```python
from build123d import *

# Parameters (mm, degrees)
SKETCH_1_W          = 42.7
SKETCH_1_H          = 33
EXTRUDE_1_DEPTH     = 4
SKETCH_2_R          = 1.5
SKETCH_2_W          = 10
SKETCH_2_H          = 4
SKETCH_2_W_2        = 4
SKETCH_2_H_2        = 14
CUT_EXTRUDE_2_DEPTH = 4


with BuildPart() as part:
    # Эскиз1 → Бобышка-Вытянуть1 (new body)
    with BuildSketch(Plane.XY):
        with Locations((17.35, 12.5)):
            Rectangle(SKETCH_1_W, SKETCH_1_H)
    extrude(amount=EXTRUDE_1_DEPTH)

    # Эскиз2 → Вырез-Вытянуть2 (cut)
    with BuildSketch(Plane.XY.offset(4)):
        with Locations((12.35, 12.5)):
            Circle(SKETCH_2_R)
        with Locations(Location((22.35, 12.5, 0), (0, 0, 180))):
            Circle(SKETCH_2_R)
        with Locations((9.85, 27)):
            Rectangle(SKETCH_2_W, SKETCH_2_H)
        with Locations((24.85, 27)):
            Rectangle(SKETCH_2_W, SKETCH_2_H)
        with Locations((-2, 3)):
            Rectangle(SKETCH_2_W_2, SKETCH_2_H_2)
        with Locations((-2, 22)):
            Rectangle(SKETCH_2_W_2, SKETCH_2_H_2)
        with Locations((24.85, -2)):
            Rectangle(SKETCH_2_W, SKETCH_2_H)
        with Locations((9.85, -2)):
            Rectangle(SKETCH_2_W, SKETCH_2_H)
        with Locations((36.7, 3)):
            Rectangle(SKETCH_2_W_2, SKETCH_2_H_2)
        with Locations((36.7, 22)):
            Rectangle(SKETCH_2_W_2, SKETCH_2_H_2)
    extrude(amount=-CUT_EXTRUDE_2_DEPTH, mode=Mode.SUBTRACT)


solid = part.part
```
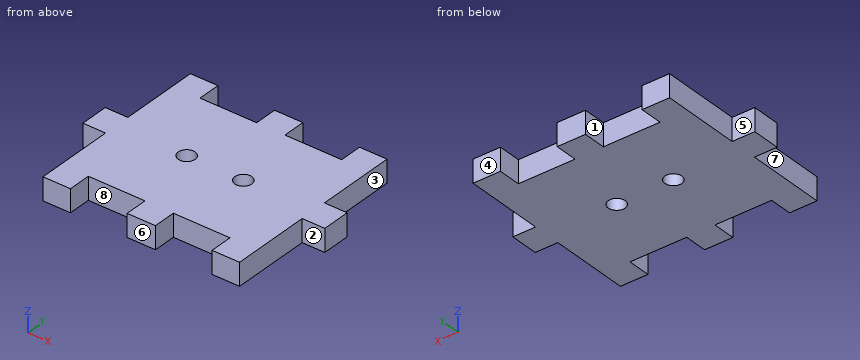
Geometry: final body of the model. Coordinates: model frame, mm. Face numbers are marked on the shaded views. A direction names the side the tool comes from. Coordinates: 2 decimals unless noted, no trailing zeros. Loops run counter-clockwise (first coordinate to the right, second up) from the corner with the lowest first, then second, coordinate; pieces in that order, holes last. Notation, with made-up numbers: (23.25, 49) -> (42.25, 49) arc R16 ccw to (42.25, 56) -> close; hole circle Ø8 at (37.25, 27.5). An arc over 180 degrees is marked (long way). Use a Markdown table: item, result. Add a question column.
(1) Pin query (flat end, axial travel): pin 1 Ø2 at (y, z) = (24.5, 2.5) entering from -X; pin 2 Ø2 at (x, z) = (24.5, 1.5) entering from -Y; pin 3 Ø1.2 at (x, z) = (25, 2) entering from +Y. Return the tip coordinate at first contact, or that it passes through.
(2) Section query D-D, the plane x = 8. Return loops of the section in (y, z), plus the area to 3 significant figures.
(3) Access query for the marked faces 4, 5, 6, 7 and 8. Directions: +Z, -Z, +X, -X, +Y, -Y. A direction counts if a zero-diameter tool reaches every point of the face in a straight line with its end or side. Return the directions, or none.
(4) Section query C-C, the plane z = 2.15. State how many separate pieces and enclosed holes the cut face has, plus the area to 3 significant figures.
(5) Mould query, pull axis X, two halves, no side actions, for the marked faces 1, 2 and 3. Classes: pulls with the +X half, pulls with the -X half, needs draft (parallel to the pull), parting line crosses it, or undercut.
(6) Section query A-A, the plane y = 12.5. Return loops of the section in (x, z), plus the area to 3 significant figures.
(7) Line query: line 1 along X through (y, z) = (26, 0.45); line 2 along Y through (x, z) = (12.35, 1.65); line 3 along Y through (x, z) = (28.5, 2). Output: solid intervals per line, ascending.
(8) Section query B-B, the plane x = 12.35. Return loops of the section in (y, z).
Answer:
| question | item | result |
|---|---|---|
| 1 | pin 1 | stops at x = 0 |
| 1 | pin 2 | stops at y = 0 |
| 1 | pin 3 | stops at y = 25 |
| 2 | outline | (0, 0) -> (25, 0) -> (25, 4) -> (0, 4) -> close |
| 2 | area | 100 mm^2 |
| 3 | face 4 | +Z, -Z, +X, -X, +Y |
| 3 | face 5 | +Z, -Z, -X, +Y |
| 3 | face 6 | +Z, -Z, +X, -X, -Y |
| 3 | face 7 | +Z, -Z, -X, -Y |
| 3 | face 8 | +Z, -Z, -Y |
| 4 | separate pieces | 1 |
| 4 | enclosed holes | 2 |
| 4 | area | 1,010 mm^2 |
| 5 | face 1 | undercut |
| 5 | face 2 | needs draft |
| 5 | face 3 | pulls with the +X half |
| 6 | outline | (-4, 0) -> (10.85, 0) -> (10.85, 4) -> (-4, 4) -> close; (13.85, 0) -> (20.85, 0) -> (20.85, 4) -> (13.85, 4) -> close; (23.85, 0) -> (38.7, 0) -> (38.7, 4) -> (23.85, 4) -> close |
| 6 | area | 147 mm^2 |
| 7 | line 1 | x = 0 to 4.85, 14.85 to 19.85, 29.85 to 34.7 |
| 7 | line 2 | y = 0 to 11, 14 to 25 |
| 7 | line 3 | y = 0 to 25 |
| 8 | outline | (0, 0) -> (11, 0) -> (11, 4) -> (0, 4) -> close; (14, 0) -> (25, 0) -> (25, 4) -> (14, 4) -> close |
